Check sheet for the modelled part. Datum: model origin and axes. Units: mm. A direction names the side the tool comes from. Round coordinates to 2 decimals unless told otherwise and drop trailing zeros. Write each loop counter-clockwise with the first axis right and the second up, starting at its lowest first coordinate (ties: lowest second). Pieces come first, ordered by that corner, then holes. Notation, with made-up numbers: (-8.5, 45.5) - (6.5, 45.5) arc R16 cw to (6.5, 59.5) - close; hole circle Ø5 at (22, 79.25). An arc over 180 degrees is marked (long way). Answer as a JSON object with one key per item and string values. Group by question number.
Item 1: Gauge pin test, flat ends, axial feed: P1, Ø7.5, axis at x = -7.5, z = -25.5, coming from the +Y side; P2, Ø1.5, axis at y = -2, z = -13.5, coming from the -X side; P3, Ø0.6, axis at x = 12, z = -22.5, coming from the -Y side. Record the tip position at first contact, or that the pin passes through.
Item 2: Sectioned sample at D-D on z = -20.25. Record the boundary of the cut face in (x, y).
Item 3: Sectioned sample at A-A on y = -5.1. Record the boundary of the cut face in (x, z), plus the area to 3 significant figures.
Item 4: Sectioned sample at B-B on x = 5.35. Record the boundary of the cut face in (y, z).
Item 5: Release check for a two-part mould opening along Y. For faces 1 (the flat face through (5, 12, -3)), 2 (the cylindrical face through (14.631, -7.407, -13.636)), 3 (the flat face through (-1, 11.3, -24)) record: pulls with the +Y half, pulls with the -Y half, needs draft (parallel to the pull), parting line crosses it, or undercut.
Item 6: Sectioned sample at C-C on x = -1.75. Record the boundary of the cut face in (y, z).
Item 7: Set-up check for faces 4 (the flat face through (-4, -11.3, -9)), 5 (the flat face through (11.514, -11.5, -9.162)), 6 (the flat face through (-3.7, -12, -24)), 7 (the flat face through (-12, 12, -23.536)): record each of +Z, -Z, +X, -X, +Y, -Y from which the full face is reachable in a straight line by a thin tool's end or side.
Item 8: Thickness scan on line 1 (Y direction, x = 3, z = -14.25); line 2 (Z direction, x = 5.35, y = 14.6). Record the ranges inside material, lowest first.
Solid Edge part; units mm, degrees
sketch "Sketch1" plane through (0, 0, 0) normal (0, 0, 1) x (1, 0, 0)
  line L0 (-11.3, -11.3) -> (11.3, -11.3)
  line L1 (11.3, -11.3) -> (11.3, 11.3)
  line L2 (11.3, 11.3) -> (-11.3, 11.3)
  line L3 (-11.3, 11.3) -> (-11.3, -11.3)
  dimension "D1" = 11.3
  dimension "D2" = 11.3
extrude "Protrusion1" add sketch "Sketch1" against normal blind 3
sketch "Sketch2" plane through (0, 0, 0) normal (0, 0, 1) x (1, 0, 0)
  line L0 (-13.3, -13.3) -> (13.3, -13.3)
  line L1 (13.3, -13.3) -> (13.3, 13.3)
  line L2 (13.3, 13.3) -> (-13.3, 13.3)
  line L3 (-13.3, 13.3) -> (-13.3, -13.3)
  line L4 (-11.3, -11.3) -> (11.3, -11.3)
  line L5 (11.3, -11.3) -> (11.3, 11.3)
  line L6 (11.3, 11.3) -> (-11.3, 11.3)
  line L7 (-11.3, 11.3) -> (-11.3, -11.3)
extrude "Extrusionsausprägung_2" add sketch "Sketch2" against normal blind 31
sketch "Sketch3" plane through (13.3, 3, -15.5) normal (1, 0, 0) x (0, -1, 0)
  circle A0 centre (8.1, -6.3) radius 5
extrude "Protrusion2" add sketch "Sketch3" along normal blind 2.7
sketch "Sketch4" plane through (16, 5.1, -9.2) normal (1, 0, 0) x (0, -1, 0)
  circle A0 centre (10.2, 0) radius 2.35
extrude "Cutout1" cut sketch "Sketch4" against normal through all
sketch "Sketch5" plane through (0, -11.3, -14) normal (0, 1, 0) x (1, 0, 0)
  line L0 (11.3, 17) -> (-3.7, 17)
  line L1 (-3.7, 3) -> (-3.7, 17)
  line L2 (-3.7, 3) -> (11.3, 3)
  line L3 (11.3, 3) -> (11.3, 17)
  dimension "D1" = 11.3
  dimension "D2" = 11.3
extrude "Cutout2" cut sketch "Sketch5" against normal through all
sketch "Sketch6" plane through (13.3, 3, -15.5) normal (1, 0, 0) x (0, -1, 0)
  line L0 (-2.3, 15.5) -> (-2.3, 2)
  line L1 (-2.3, 2) -> (-5.3, 2)
  line L2 (-5.3, 2) -> (-5.3, 15.5)
  line L3 (-5.3, 15.5) -> (-2.3, 15.5)
  dimension "D1" = 2.3
extrude "Cutout3" cut sketch "Sketch6" against normal up to next
sketch "Sketch7" plane through (-4.5, 12.3, -18.5) normal (0, 0, -1) x (-1, 0, 0)
  line L0 (8.8, 1) -> (-17.8, 1)
  line L1 (-17.8, 1) -> (-17.8, -25.6)
  line L2 (-17.8, -25.6) -> (8.8, -25.6)
  line L3 (8.8, -25.6) -> (8.8, 1)
extrude "Extrusionsausprägung_5" add sketch "Sketch7" against normal blind 3
sketch "Sketch8" plane through (-13.3, 0, -15.5) normal (-1, 0, 0) x (0, 1, 0)
  line L0 (13.3, -15.5) -> (-13.3, -15.5)
  line L1 (-13.3, -15.5) -> (-13.3, -12.5)
  line L2 (-13.3, -12.5) -> (13.3, -12.5)
  line L3 (13.3, -12.5) -> (13.3, -15.5)
  dimension "D1" = 13.3
extrude "Cutout4" cut sketch "Sketch8" against normal through all
sketch "Sketch9" plane through (0, 0, -3) normal (0, 0, 1) x (0, -1, 0)
  line L0 (11.3, -13.3) -> (11.3, -11.3)
  line L1 (11.3, -11.3) -> (-3.7, -11.3)
  line L2 (-3.7, -11.3) -> (-3.7, -13.3)
  line L3 (-3.7, -13.3) -> (11.3, -13.3)
  dimension "D1" = 11.3
  dimension "D2" = 11.3
extrude "Cutout5" cut sketch "Sketch9" against normal up to vertex (12.5 mm away)
sketch "Sketch10" plane through (0, 13.3, -17) normal (0, 1, 0) x (0, 0, 1)
  circle A0 centre (-6.65, 5.35) radius 6
extrude "Extrusionsausprägung_6" add sketch "Sketch10" along normal blind 3
sketch "Sketch11" plane through (4.9, 16.3, -24.7) normal (0, 1, 0) x (1, 0, 0)
  circle A0 centre (0.45, -1.05) radius 2.35
extrude "Cutout6" cut sketch "Sketch11" against normal up to next
sketch "Sketch12" plane through (0, 13.3, -18) normal (0, 1, 0) x (1, 0, 0)
  line L0 (-11.3, 13) -> (-13.3, 5.5359)
  line L1 (-13.3, 13) -> (-13.3, 5.5359)
  line L2 (-11.3, 13) -> (-13.3, 13)
  dimension "D1" = 11.3
extrude "Cutout7" cut sketch "Sketch12" against normal up to next
sketch "Sketch13" plane through (0.3352, -13.3, -18) normal (0, -1, 0) x (1, 0, 0)
  line L0 (2.9648, 2.5) -> (7.9648, 2.5)
  line L1 (7.9648, 2.5) -> (7.9648, 15)
  line L2 (7.9648, 15) -> (2.9648, 15)
  line L3 (2.9648, 15) -> (2.9648, 2.5)
  dimension "D1" = 2.9648
extrude "Cutout8" cut sketch "Sketch13" against normal up to next
sketch "Sketch14" plane through (-12.3, 7.5, -3) normal (0, 0, 1) x (0, 1, 0)
  line L0 (2.8, -1) -> (3.5071, -0.2929)
  line L1 (3.5071, -0.2929) -> (4.5071, -1.2929)
  line L2 (4.5071, -1.2929) -> (3.8, -2)
  line L3 (3.8, -2) -> (3.8, -1)
  line L4 (3.8, -1) -> (2.8, -1)
  dimension "D1" = 3.8
  dimension "D2" = 2.8
extrude "Cutout9" cut sketch "Sketch14" against normal up to vertex (12.5 mm away)
mirror "Mirror1" about plane through (0, 0, 0) normal (1, 0, 0) of "Cutout9"
mirror "Mirror2" about plane through (0, 0, 0) normal (0, -1, 0) of "Cutout9", "Mirror1"
sketch "Sketch15" plane through (0, 12.3, -31) normal (0, 0, -1) x (-1, 0, 0)
  line L0 (11.3, -1) -> (13.3, -1)
  line L1 (13.3, -1) -> (13.3, -23.6)
  line L2 (13.3, -23.6) -> (11.3, -23.6)
  line L3 (11.3, -23.6) -> (11.3, -1)
extrude "Cutout10" cut sketch "Sketch15" against normal blind 7.5
chamfer "Fase_5" distance 0.5 angle 45 2 edges at (3, 16.3, -23.65) (16, -2.75, -9.2)
fillet "Verrundung_6" radius 2 4 edges at (13.3, 13.3, -17) (13.3, -13.3, -17) (-13.3, 13.3, -13.2679) (-13.3, -13.3, -13.2679)
sketch "Sketch16" plane through (0, -13.3, -17) normal (0, -1, 0) x (1, 0, 0)
  line L0 (-13.3, -6.5359) -> (-11.3, -6.5359)
  line L1 (-11.3, -6.5359) -> (-11.3, -14)
  line L2 (-11.3, -14) -> (-13.3, -6.5359)
extrude "Cutout11" cut sketch "Sketch16" against normal through all
sketch "Sketch17" plane through (12.3, -4, -31) normal (0, 0, -1) x (0, 1, 0)
  line L0 (-9.3, -1) -> (9.3, -1)
  line L1 (9.3, -1) -> (9.3, 1)
  line L2 (9.3, 1) -> (12.3, 1)
  line L3 (12.3, 1) -> (12.3, -1)
  line L4 (12.3, -1) -> (15.3, -1)
  line L5 (15.3, -1) -> (15.3, -23.6)
  line L6 (15.3, -23.6) -> (-7.3, -23.6)
  line L7 (-7.3, -23.6) -> (-7.3, -16)
  line L8 (-7.3, -16) -> (-9.3, -16)
  line L9 (-9.3, -16) -> (-9.3, -1)
extrude "Extrusionsausschnitt_21" cut sketch "Sketch17" against normal blind 13.5
sketch "Sketch18" plane through (12.3, -4, -31) normal (0, 0, -1) x (0, 1, 0)
  line L0 (-24.7024, -32.1956) -> (31.7056, -32.1956)
  line L1 (31.7056, -32.1956) -> (31.7056, 6.9175)
  line L2 (31.7056, 6.9175) -> (-24.7024, 6.9175)
  line L3 (-24.7024, 6.9175) -> (-24.7024, -32.1956)
extrude "Extrusionsausschnitt_22" cut sketch "Sketch18" against normal blind 1
properties material "Nylon, allgemein"
Completed:
{
 "1": {"P1": "y = 13.3", "P2": "x = 11.3", "P3": "y = -13.26"},
 "2": {"outline": "(-13.3, -11.3) arc R2 ccw to (-11.3, -13.3) - (-3.7, -13.3) - (-3.7, -11.3) - (-11.3, -11.3) - (-11.3, 11.3) - (11.3, 11.3) - (11.3, 8.3) - (13.3, 8.3) - (13.3, 11.3) arc R2 ccw to (11.3, 13.3) - (10.29, 13.3) - (10.29, 16.3) - (0.41, 16.3) - (0.41, 13.3) - (-11.3, 13.3) arc R2 ccw to (-13.3, 11.3) - close; (11.3, -13.3) arc R2 ccw to (13.3, -11.3) - (13.3, 5.3) - (11.3, 5.3) - close"},
 "3": {"outline": "(-13.3, -23.5) - (-11.3, -23.5) - (-11.3, -17.5) - (11.3, -17.5) - (11.3, -30) - (13.3, -30) - (13.3, -14.2) - (16, -14.2) - (16, -12.05) - (15.5, -11.55) - (11.3, -11.55) - (11.3, -15.5) - (-13.3, -15.5) - close; (11.3, -6.85) - (15.5, -6.85) - (16, -6.35) - (16, -4.2) - (13.3, -4.2) - (13.3, -3) - (11.3, -3) - close", "area": "120 mm²"},
 "4": {"outline": "(-13.3, -17.5) - (11.3, -17.5) - (11.3, -21.3) - (15.8, -21.3) - (16.3, -20.8) - (16.3, -17.65) - (13.3, -17.65) - (13.3, -3) - (11.3, -3) - (11.3, -15.5) - (-13.3, -15.5) - close; (11.3, -30) - (13.3, -30) - (13.3, -29.65) - (16.3, -29.65) - (16.3, -26.5) - (15.8, -26) - (11.3, -26) - close"},
 "5": {"face 1": "needs draft", "face 2": "parting line crosses it", "face 3": "undercut"},
 "6": {"outline": "(-13.3, -17.5) - (11.3, -17.5) - (11.3, -30) - (13.3, -30) - (13.3, -3) - (11.3, -3) - (11.3, -15.5) - (-11.3, -15.5) - (-11.3, -3) - (-13.3, -3) - close"},
 "7": {"face 4": "+Z, -X", "face 5": "+Z", "face 6": "-Z, -Y", "face 7": "-Z, -X, +Y, -Y"},
 "8": {"line 1": "-13.3 to -11.3, 11.3 to 13.3", "line 2": "-29.65 to -26, -21.3 to -17.65"}
}
